Can you work these out from the drawing? Everything is in mm from the part's minimum corner. A direction names the side the tool comes from. Coordinates: 2 decimals unless noted, no trailing zeros. Order: outer loops, then holes, each group sorted by start corner. A loop starts at its lowest first (then second) coordinate and runs counter-clockwise, first axis right, second up. Notation, with made-up numbers: (58, 20.5) -> (92, 20.5) arc R23 ccw to (92, 39.5) -> close; hole circle Ø8 at (86, 26.25). An arc over 180 degrees is marked (long way). Use a Markdown table: item, result. Add a question column.
1) If we section it at A-A (y = 16): Write out the boundary of the cut face in (x, z).
2) If we section it at C-C (z = 3.75): Write out the boundary of the cut face in (x, y), plus the area to 4 significant figures.
3) If we section it at D-D (z = 11): Write out the boundary of the cut face in (x, y).
4) If I drill on L1, parallel to X at y = 15, z = 8.75; L2, parallel to X at y = 16, z = 3.6; L3, parallel to Y at x = 16, z = 1.2, over which ranges is the centre line in solid material (lowest first)? Write a range as [from, to].
5) Which directions (+Z, -Z, +X, -X, +Y, -Y) give clear straight access to the entire face, cutting with the end or side of a thin tool? Please do the marked faces 1 and 2.
6) Will these pins go through, and if not, where does the flat tip stop? pin 1 Ø6 at (x, y) = (12, 20.5) entering from -Z; pin 2 Ø8 at (x, z) = (26, 6.5) entering from +Y; pin 3 Ø3 at (x, y) = (16, 16) entering from -Z; pin 4 Ø4 at (y, z) = (4.5, 2) entering from +X.
7) Thinking about a two-plate mould opening in Y: for the marked faces 3, 4 and 5, which applies, +Y half, -Y half, draft (parallel to the pull), parting line (faces both ways), or undercut?
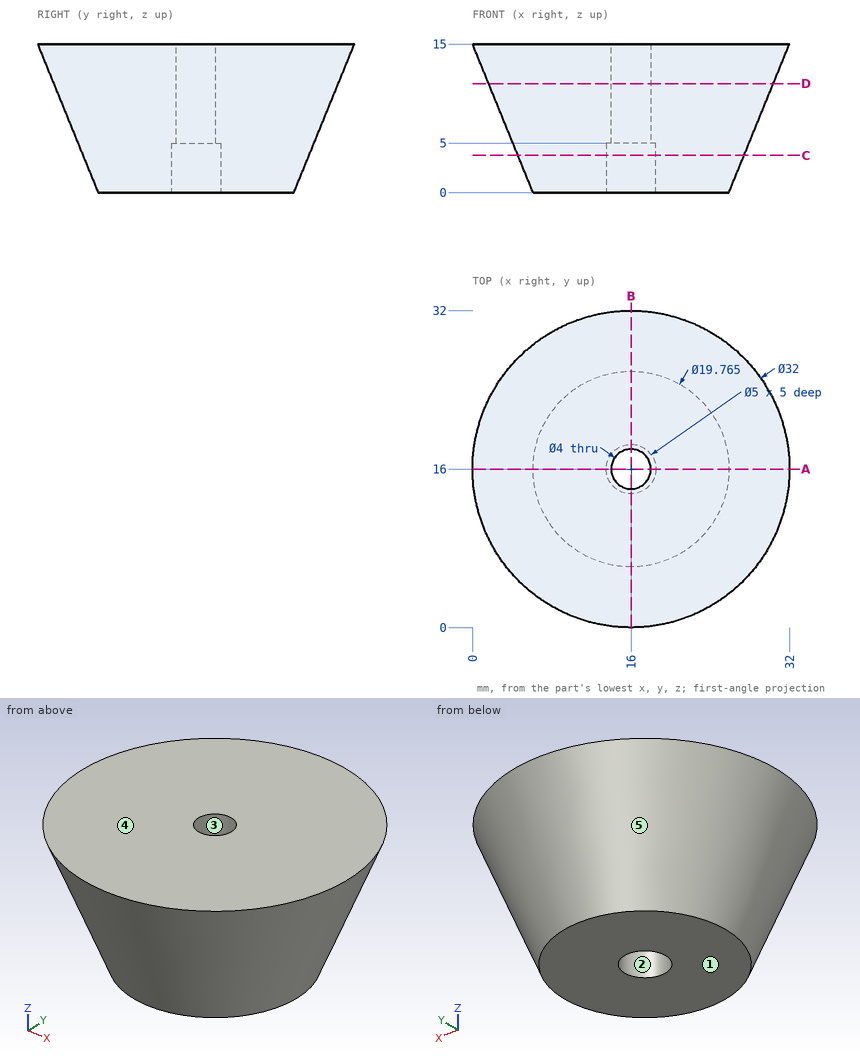
Answer sheet:
| question | item | result |
|---|---|---|
| 1 | outline | (0, 15) -> (6.12, 0) -> (13.5, 0) -> (13.5, 5) -> (14, 5) -> (14, 15) -> close; (18, 5) -> (18.5, 5) -> (18.5, 0) -> (25.88, 0) -> (32, 15) -> (18, 15) -> close |
| 2 | outline | circle Ø22.82 at (16, 16); hole circle Ø5 at (16, 16) |
| 2 | area | 389.5 mm2 |
| 3 | outline | circle Ø28.74 at (16, 16); hole circle Ø4 at (16, 16) |
| 4 | L1 | [2.59, 14.27], [17.73, 29.41] |
| 4 | L2 | [4.65, 13.5], [18.5, 27.35] |
| 4 | L3 | [5.63, 13.5], [18.5, 26.37] |
| 5 | face 1 | -Z, +X, -X, +Y, -Y |
| 5 | face 2 | -Z |
| 6 | pin 1 | z = 0 |
| 6 | pin 2 | y = 27.68 |
| 6 | pin 3 | through |
| 6 | pin 4 | x = 21.3 |
| 7 | face 3 | undercut |
| 7 | face 4 | draft |
| 7 | face 5 | parting line |
